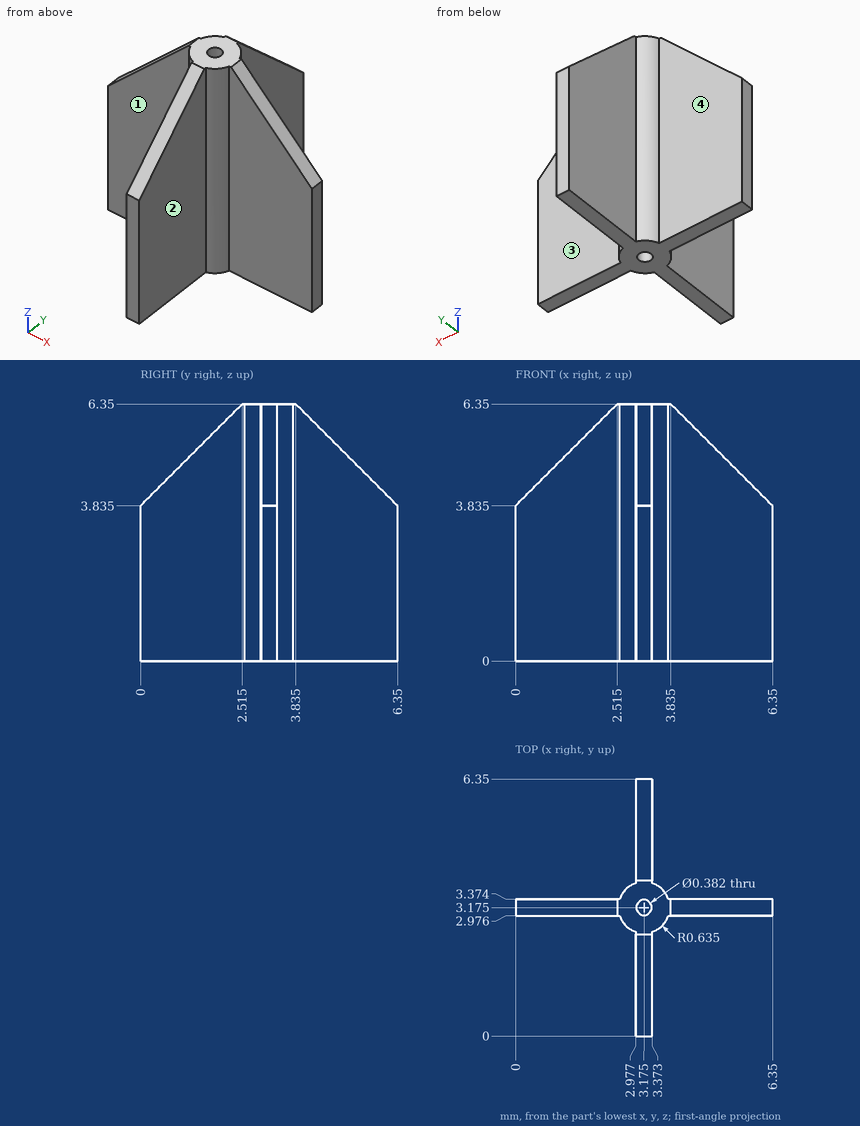
For this review, use the dimensioned drawing (mm, ordinates from the lowest corner) and the shaded views. A direction names the side the tool comes from. Coordinates: 2 decimals unless noted, no trailing zeros. Use a Markdown table: item, result. Add a question column.
1. To check wall thickness, follow line 1 (Y direction, x = 1, z = 4.25) (1 decimal); line 2 (X direction, y = 4.25, z = 4.75); line 3 (X direction, y = 2.75, z = 2.5) (1 decimal). State the ranges of each line that lie inside material, in increasing order.
2. Machinability: for the marked faces 1, 2, 3 and 4, which of the approach directions +Z, -Z, +X, -X, +Y, -Y give a long, thin tool a straight path to every point of the face, cutting with its end or side? Answer none if there is none.
3. Clearance check with flat-ended pins moving along their axes: pin 1 Ø1 at (x, z) = (4.5, 3) entering from -Y; pin 2 Ø0.8 at (x, z) = (1.5, 3.5) entering from +Y; pin 3 Ø1 at (y, z) = (5.5, 3) entering from +X. State where each tip first meets the part, or that it passes through.
Returned:
| question | item | result |
|---|---|---|
| 1 | line 1 | y = 3 to 3.4 |
| 1 | line 2 | x = 2.98 to 3.37 |
| 1 | line 3 | x = 2.7 to 3.6 |
| 2 | face 1 | +Z, -Z, -X, -Y |
| 2 | face 2 | +Z, -Z, +X, -Y |
| 2 | face 3 | +Z, -Z, +X, +Y |
| 2 | face 4 | +Z, -Z, -X, +Y |
| 3 | pin 1 | stops at y = 2.98 |
| 3 | pin 2 | stops at y = 3.37 |
| 3 | pin 3 | stops at x = 3.37 |
